Check sheet for the drawn part. Datum: minimum x, y, z corner. Units: mm. A direction names the side the tool comes from. Round coordinates to 2 decimals unless told otherwise and drop trailing zeros. Order: outer loops, then holes, each group sorted by start corner. A loop starts at its lowest first (then second) coordinate and runs counter-clockwise, first axis right, second up. Notation, with made-up numbers: (11, 55) -> (36, 55) arc R22 ccw to (36, 85) -> close; hole circle Ø5 at (-19, 58.25). An arc over 180 degrees is marked (long way). Answer in a Markdown table with one row per item.
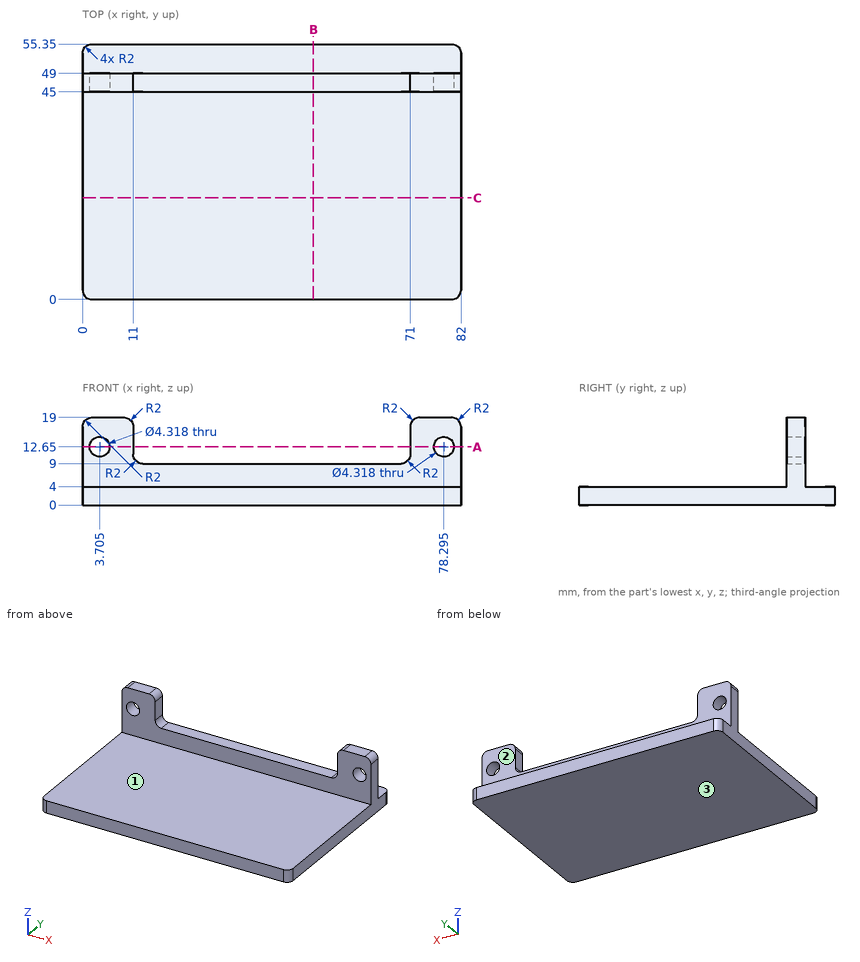
(1) Section check B-B on x = 50. Record the boundary of the cut face in (y, z).
Solutions:
| item | result |
|---|---|
| outline | (0, 0) -> (55.35, 0) -> (55.35, 4) -> (49, 4) -> (49, 9) -> (45, 9) -> (45, 4) -> (0, 4) -> close |
(2) Section check C-C on y = 22. Record the boundary of the cut face in (x, z), plus the area to 3 significant figures.
Solutions:
| item | result |
|---|---|
| outline | (0, 0) -> (82, 0) -> (82, 4) -> (0, 4) -> close |
| area | 328 mm^2 |
(3) Tool access check on the marked faces 1, 2 and 3. Record the directions out of +Z, -Z, +X, -X, +Y, -Y that give a thin tool (end or side, any length) a straight path to the whole face; none if there is none.
Solutions:
| item | result |
|---|---|
| face 1 | +Z, +X, -X, -Y |
| face 2 | +Z, +X, -X, +Y |
| face 3 | -Z, +X, -X, +Y, -Y |
(4) Depth check by flat-ended pin: pin 1 Ø4.5 at (x, z) = (26.5, 11) entering from +Y; pin 2 Ø2 at (x, y) = (64.5, 41) entering from +Z; pin 3 Ø2 at (x, z) = (67.5, 11) entering from -Y; pin 4 Ø4.5 at (x, y) = (47, 47) entering from +Z. Enter the tip coordinate at first touch or a pass-through.
Solutions:
| item | result |
|---|---|
| pin 1 | y = 49 |
| pin 2 | z = 4 |
| pin 3 | through |
| pin 4 | z = 9 |
(5) Section check A-A on z = 12.65. Record the boundary of the cut face in (x, y).
Solutions:
| item | result |
|---|---|
| outline | (0, 45) -> (1.55, 45) -> (1.55, 49) -> (0, 49) -> close; (5.86, 45) -> (11, 45) -> (11, 49) -> (5.86, 49) -> close; (71, 45) -> (76.14, 45) -> (76.14, 49) -> (71, 49) -> close; (80.45, 45) -> (82, 45) -> (82, 49) -> (80.45, 49) -> close |
(6) Scan lines: probe 1 along X at (y, z) = (47.45, 12.65); probe 2 along Z at (x, y) = (38.5, 45.5); probe 3 along Y at (x, z) = (68, 6.75). Record each from-to range of solid material in increasing order. Write a range as from..to.
Solutions:
| item | result |
|---|---|
| probe 1 | 0..1.55, 5.86..11, 71..76.14, 80.45..82 |
| probe 2 | 0..9 |
| probe 3 | 45..49 |
